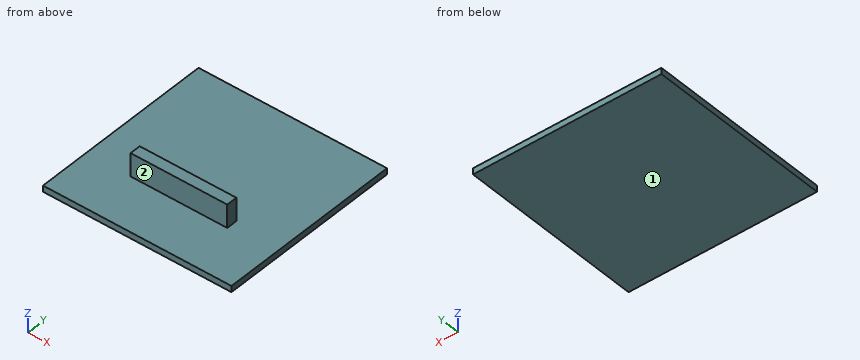
from build123d import *

# Parameters (mm, degrees)
F0_W      = 762
F0_H      = 762
F1_DEPTH  = 25.4
F1_FACE_W = 762
F1_FACE_H = 25.4
F2_DEPTH  = 12.7
F4_W      = 397.13651
F4_H      = 44.45
F5_DEPTH  = 95.25


with BuildPart() as f1:
    # F0 (on Top) → F1 (new body)
    with BuildSketch(Plane.XY):
        Rectangle(F0_W, F0_H)
    extrude(amount=F1_DEPTH)

    # F1_face (on face) → F2 (join)
    with BuildSketch(Plane(origin=(381, 0, 12.7), x_dir=(0, 1, 0), z_dir=(1, 0, 0))):
        Rectangle(F1_FACE_W, F1_FACE_H)
    extrude(amount=F2_DEPTH)

    # F4 (on face) → F5 (join)
    with BuildSketch(Plane.XY.offset(25.4)):
        with Locations((0, -146.924108)):
            Rectangle(F4_W, F4_H)
    extrude(amount=F5_DEPTH)


solid = f1.part
Check sheet for the modelled part. Datum: model origin and axes. Units: mm. Face numbers are marked on the shaded views. A direction names the side the tool comes from. Give positions to 0.01 mm unless a question says otherwise; leave off trailing zeros. Write each loop counter-clockwise with the first axis right and the second up, starting at its lowest first coordinate (ties: lowest second). Pieces come first, ordered by that corner, then holes. Notation, with made-up numbers: M 18,87 L 66,87 A22 ccw 66,116 Z; hole C 74.5,-11 d4. An arc over 180 degrees is marked long. Use one line per item in the form item = value.
(1) Section check A-A on x = -114. Record the boundary of the cut face in (y, z).
Answer block:
outline = M -381,0 L 381,0 L 381,25.4 L -124.7,25.4 L -124.7,120.65 L -169.15,120.65 L -169.15,25.4 L -381,25.4 Z
(2) Material ranges on line 1 along Z through (x, y) = (-126.5, 133.5); line 2 along Y through (x, z) = (108, 91.5); line 3 along X through (y, z) = (-132, 98.5), recorded low to high.
Answer block:
line_1 = 0 to 25.4
line_2 = -169.15 to -124.7
line_3 = -198.57 to 198.57
(3) Depth check by flat-ended pin: P1, Ø10, axis at x = 41.5, z = 53.5, coming from the -Y side; P2, Ø13.5, axis at y = -144.5, z = 82, coming from the -X side; P3, Ø3, axis at y = 20.5, z = 26.5, coming from the +X side; P4, Ø6, axis at x = -29, y = -246, coming from the +Z side. Enter the tip coordinate at first touch or a pass-through.
Answer block:
P1 = -169.15
P2 = -198.57
P3 = 393.7
P4 = 25.4
(4) Section check C-C on y = 46. Record the boundary of the cut face in (x, z), plus the area to 3 significant figures.
Answer block:
outline = M -381,0 L 393.7,0 L 393.7,25.4 L -381,25.4 Z
area = 19,700 mm2
(5) Tool access check on the marked faces 1 and 2. Record the directions out of +Z, -Z, +X, -X, +Y, -Y that give a thin tool (end or side, any length) a straight path to the whole face; none if there is none.
Answer block:
face_1 = -Z, +X, -X, +Y, -Y
face_2 = +Z, +X, -X, -Y
(6) Section check B-B on z = 77. Record the boundary of the cut face in (x, y), plus the area to 3 significant figures.
Answer block:
outline = M -198.57,-169.15 L 198.57,-169.15 L 198.57,-124.7 L -198.57,-124.7 Z
area = 17,700 mm2
